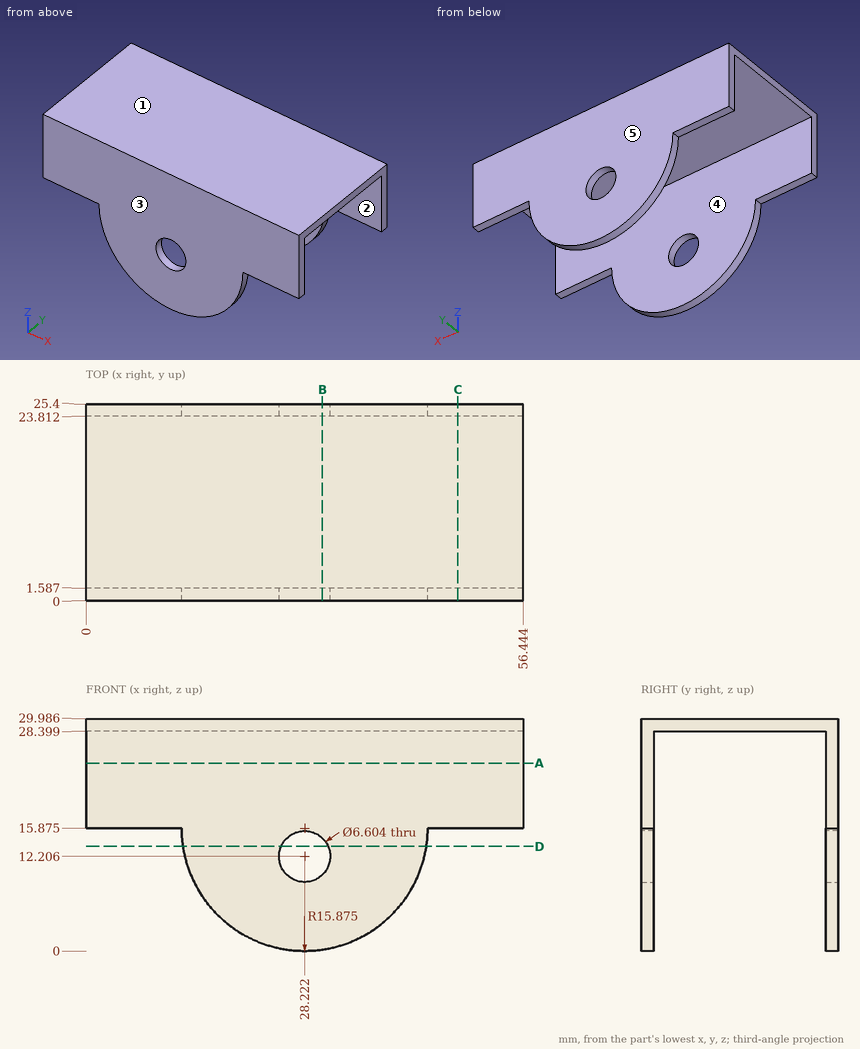
Geometry: see drawing. Coordinates: mm, zero at the bounding-box minimum. A direction names the side the tool comes from. Round coordinates to 2 decimals unless told otherwise and drop trailing zeros. Order: outer loops, then holes, each group sorted by start corner. A loop starts at its lowest first (then second) coordinate and runs counter-clockwise, first axis right, second up. Notation, with made-up numbers: (67.25, 16.25) - (110.25, 16.25) arc R8 ccw to (110.25, 31.25) - close; hole circle Ø7 at (-27.5, -4). An arc over 180 degrees is marked (long way). Use a Markdown table: item, result. Add a question column.
1. Line query: probe 1 along Y at (x, z) = (32, 9.5); probe 2 along Z at (x, y) = (6, 5.5). Output: solid intervals per line, ascending.
2. Section query C-C (x = 48). Return the cut outline in (y, z) (1 decimal).
3. Section query D-D (z = 13.5). Return the cut outline in (x, y) (1 decimal).
4. Section query A-A (z = 24.25). Return the cut outline in (x, y) (1 decimal).
5. Mould query, pull axis Y, two halves, no side actions, for the marked faces 3, 4 and 5. Classes: +Y half, -Y half, draft (parallel to the pull), parting line (faces both ways), or undercut.
6. Section query B-B (x = 30.5). Return the cut outline in (y, z) (1 decimal), then the cut area to 3 significant figures.
7. Set-up query: the marked faces 1 and 2. Return all of +Z, -Z, +X, -X, +Y, -Y with unobstructed straight access to the full face (end or side cutting, diameter ignored); none if empty.
8. First-contact query: pin 1 (5 mm diameter, centred on y = 23, z = 9.5, fed in from +X); pin 2 (0.8 mm diameter, centred on x = 51.5, y = 24.5, fed in from -Z) (1 decimal); pin 3 (8 mm diameter, centred on y = 20, z = 10, fed in from -X). Flat tips, straight axial feed; report the tip coordinate or a pass-through.
Derived:
| question | item | result |
|---|---|---|
| 1 | probe 1 | 0 to 1.59, 23.81 to 25.4 |
| 1 | probe 2 | 28.4 to 29.99 |
| 2 | outline | (0, 15.9) - (1.6, 15.9) - (1.6, 28.4) - (23.8, 28.4) - (23.8, 15.9) - (25.4, 15.9) - (25.4, 30) - (0, 30) - close |
| 3 | outline | (12.5, 0) - (25.2, 0) - (25.2, 1.6) - (12.5, 1.6) - close; (12.5, 23.8) - (25.2, 23.8) - (25.2, 25.4) - (12.5, 25.4) - close; (31.3, 0) - (43.9, 0) - (43.9, 1.6) - (31.3, 1.6) - close; (31.3, 23.8) - (43.9, 23.8) - (43.9, 25.4) - (31.3, 25.4) - close |
| 4 | outline | (0, 0) - (56.4, 0) - (56.4, 1.6) - (0, 1.6) - close; (0, 23.8) - (56.4, 23.8) - (56.4, 25.4) - (0, 25.4) - close |
| 5 | face 3 | -Y half |
| 5 | face 4 | undercut |
| 5 | face 5 | +Y half |
| 6 | outline | (0, 0.2) - (1.6, 0.2) - (1.6, 9.8) - (0, 9.8) - close; (0, 14.6) - (1.6, 14.6) - (1.6, 28.4) - (23.8, 28.4) - (23.8, 14.6) - (25.4, 14.6) - (25.4, 30) - (0, 30) - close; (23.8, 0.2) - (25.4, 0.2) - (25.4, 9.8) - (23.8, 9.8) - close |
| 6 | area | 115 mm2 |
| 7 | face 1 | +Z, +X, -X, +Y, -Y |
| 7 | face 2 | -Z, +X, -X |
| 8 | pin 1 | x = 43.58 |
| 8 | pin 2 | z = 15.9 |
| 8 | pin 3 | x = 13.05 |
